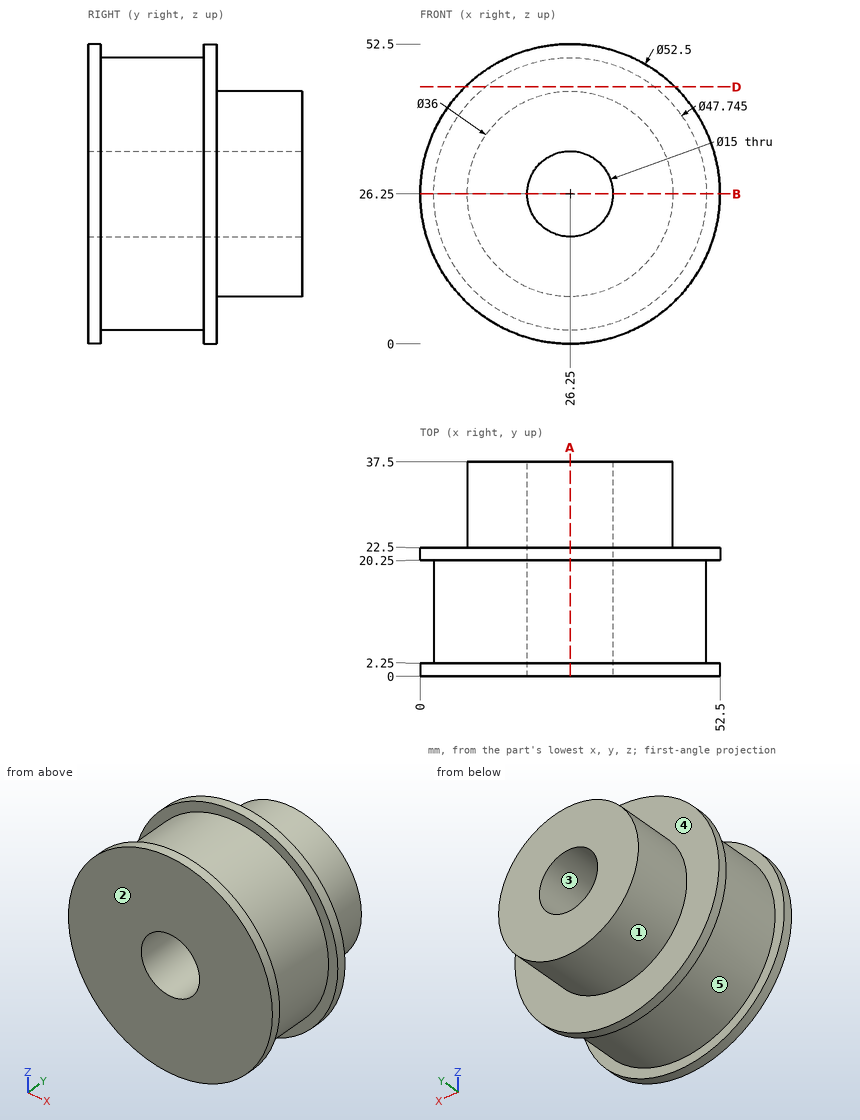
Drawing for the job (mm, zero at the part's lowest x, y, z). A direction names the side the tool comes from. Give positions to 0.01 mm unless a question says otherwise; leave off trailing zeros. Write each loop counter-clockwise with the first axis right and the second up, starting at its lowest first coordinate (ties: lowest second). Pieces come first, ordered by that corner, then holes. Notation, with made-up numbers: (0.5, 72) - (23.5, 72) arc R35 cw to (23.5, 104) - close; hole circle Ø2 at (49, 19). An arc over 180 degrees is marked (long way). Answer as CSV lines item,"result".
Q1. Band-saw the part on A-A (x = 26.25). Give the cut face in (y, z), and give its area (3 significant figures).
Result set:
outline,"(0, 0) - (2.25, 0) - (2.25, 2.38) - (20.25, 2.38) - (20.25, 0) - (22.5, 0) - (22.5, 8.25) - (37.5, 8.25) - (37.5, 18.75) - (0, 18.75) - close; (0, 33.75) - (37.5, 33.75) - (37.5, 44.25) - (22.5, 44.25) - (22.5, 52.5) - (20.25, 52.5) - (20.25, 50.12) - (2.25, 50.12) - (2.25, 52.5) - (0, 52.5) - close"
area,"1,070 mm²"
Q2. Band-saw the part on D-D (z = 45). Give the cut face in (x, y).
Result set:
outline,"(7.88, 0) - (44.62, 0) - (44.62, 2.25) - (41.03, 2.25) - (41.03, 20.25) - (44.62, 20.25) - (44.62, 22.5) - (7.88, 22.5) - (7.88, 20.25) - (11.47, 20.25) - (11.47, 2.25) - (7.88, 2.25) - close"
Q3. 3-axis set-ups, long thin cutter, end or side, ignore diameter. For the marked faces 1 and 2: which of +Z, -Z, +X, -X, +Y, -Y reach the whole face in a straight line?
Result set:
face 1,"+Y"
face 2,"+Z, -Z, +X, -X, -Y"
Q4. Flat gauge pins, fed straight in: pin 1 Ø3 at (x, y) = (26, 28) entering from -Z; pin 2 Ø4 at (x, z) = (7, 17) entering from +Y; pin 3 Ø1 at (y, z) = (21.5, 25.5) entering from +X. Where does each tip first touch, or does it go through?
Result set:
pin 1,"z = 8.25"
pin 2,"y = 22.5"
pin 3,"x = 52.5"
Q5. Drill centre lines: line 1 (Z direction, x = 26, y = 10); line 2 (X direction, y = 29, z = 26.25). Where is each one in solid material? Low to high. Write a range as from..to.
Result set:
line 1,"2.38..18.75, 33.75..50.12"
line 2,"8.25..18.75, 33.75..44.25"
Q6. Pull direction Z, two halves, no side cores. Call the marked faces 3, 4 and 5: released by +Z, released by -Z, zero draft, split by the parting line, or undercut.
Result set:
face 3,"undercut"
face 4,"zero draft"
face 5,"split by the parting line"
Q7. Band-saw the part on B-B (z = 26.25). Give the cut face in (x, y).
Result set:
outline,"(0, 0) - (18.75, 0) - (18.75, 37.5) - (8.25, 37.5) - (8.25, 22.5) - (0, 22.5) - (0, 20.25) - (2.38, 20.25) - (2.38, 2.25) - (0, 2.25) - close; (33.75, 0) - (52.5, 0) - (52.5, 2.25) - (50.12, 2.25) - (50.12, 20.25) - (52.5, 20.25) - (52.5, 22.5) - (44.25, 22.5) - (44.25, 37.5) - (33.75, 37.5) - close"
